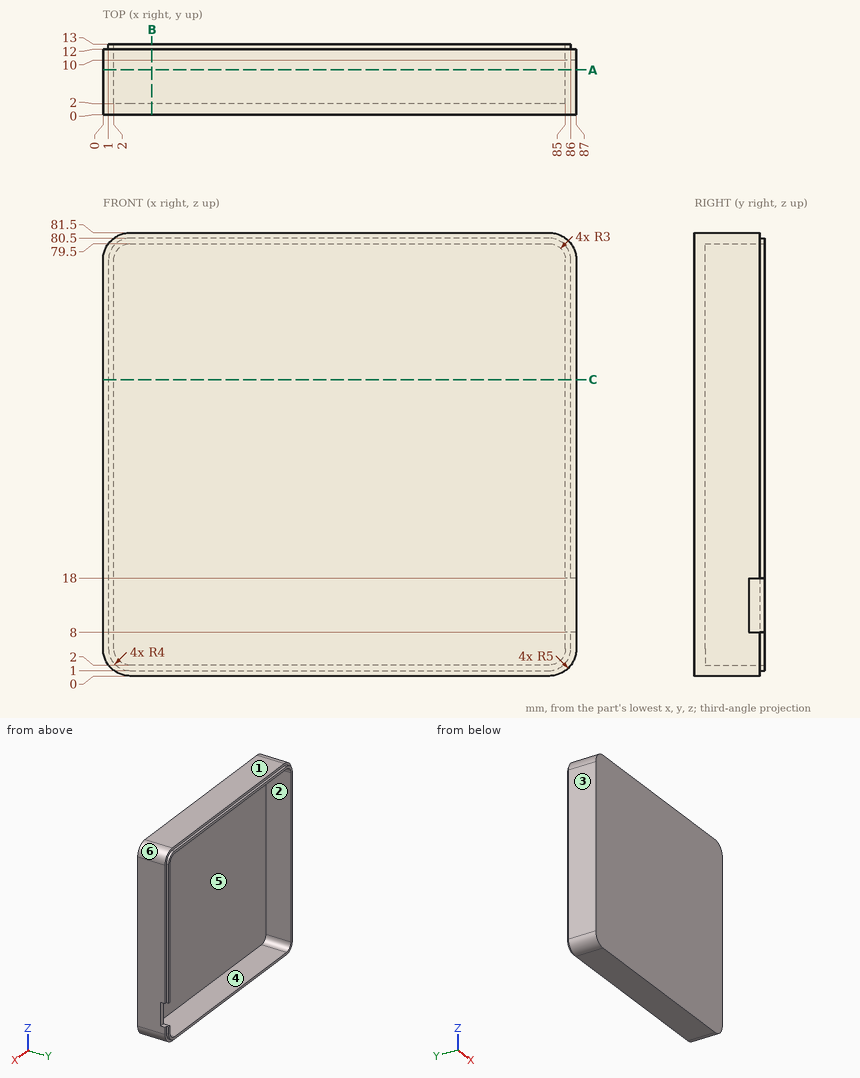
Geometry: see drawing. Coordinates: mm, zero at the bounding-box minimum. A direction names the side the tool comes from. Coordinates: 2 decimals unless noted, no trailing zeros. Order: outer loops, then holes, each group sorted by start corner. A loop starts at its lowest first (then second) coordinate and runs counter-clockwise, first axis right, second up. Notation, with made-up numbers: (73, 59) -> (121, 59) arc R36 ccw to (121, 96) -> close; hole circle Ø11 at (-26.5, 30.25). An arc over 180 degrees is marked (long way). Write each question's results on one line, items separated by ' | '. Start each with the question number.
1) Set-up query: the marked faces 5 and 6. Return all of +Z, -Z, +X, -X, +Y, -Y with unobstructed straight access to the full face (end or side cutting, diameter ignored); none if empty.
2) Cut plane C-C, the plane z = 54.5. Output: boundary loops of the cut face in (x, y), and give its area (3 significant figures).
3) First-contact query: pin 1 (23 mm diameter, centred on x = 45, z = 34, fed in from +Y); pin 2 (0.8 mm diameter, centred on x = 33, y = 12.5, fed in from +Z); pin 3 (2 mm diameter, centred on x = 85.5, y = 11, fed in from -Z). Flat tips, straight axial feed; report the tip coordinate or a pass-through.
4) Mould query, pull axis Z, two halves, no side actions, for the marked faces 1, 2, 3 and 4. Classes: released by +Z, released by -Z, zero draft, split by the parting line, or undercut.
5) Cut plane A-A, the plane y = 8.25. Output: boundary loops of the cut face in (x, z), and give its area (3 significant figures).
6) Material intervals for line 1 along X through (y, z) = (4.5, 55); line 2 along Z through (x, y) = (27.5, 6); line 3 along Z through (x, y) = (75.5, 12.25), sorted ascending.
7) Cut plane B-B, the plane x = 9. Output: boundary loops of the cut face in (y, z).
Checks:
1) face 5: +Y | face 6: +Z, +X, +Y, -Y
2) outline: (0, 0) -> (87, 0) -> (87, 12) -> (86, 12) -> (86, 13) -> (85, 13) -> (85, 2) -> (2, 2) -> (2, 13) -> (1, 13) -> (1, 12) -> (0, 12) -> close | area: 216 mm^2
3) pin 1: y = 2 | pin 2: z = 80.5 | pin 3: z = 0.67
4) face 1: released by +Z | face 2: undercut | face 3: zero draft | face 4: undercut
5) outline: (0, 5) arc R5 ccw to (5, 0) -> (82, 0) arc R5 ccw to (87, 5) -> (87, 76.5) arc R5 ccw to (82, 81.5) -> (5, 81.5) arc R5 ccw to (0, 76.5) -> close; hole (2, 5) arc R3 ccw to (5, 2) -> (82, 2) arc R3 ccw to (85, 5) -> (85, 76.5) arc R3 ccw to (82, 79.5) -> (5, 79.5) arc R3 ccw to (2, 76.5) -> close | area: 644 mm^2
6) line 1: 0 to 2, 85 to 87 | line 2: 0 to 2, 79.5 to 81.5 | line 3: 1 to 2, 79.5 to 80.5
7) outline: (0, 0) -> (12, 0) -> (12, 1) -> (13, 1) -> (13, 2) -> (2, 2) -> (2, 79.5) -> (13, 79.5) -> (13, 80.5) -> (12, 80.5) -> (12, 81.5) -> (0, 81.5) -> close
